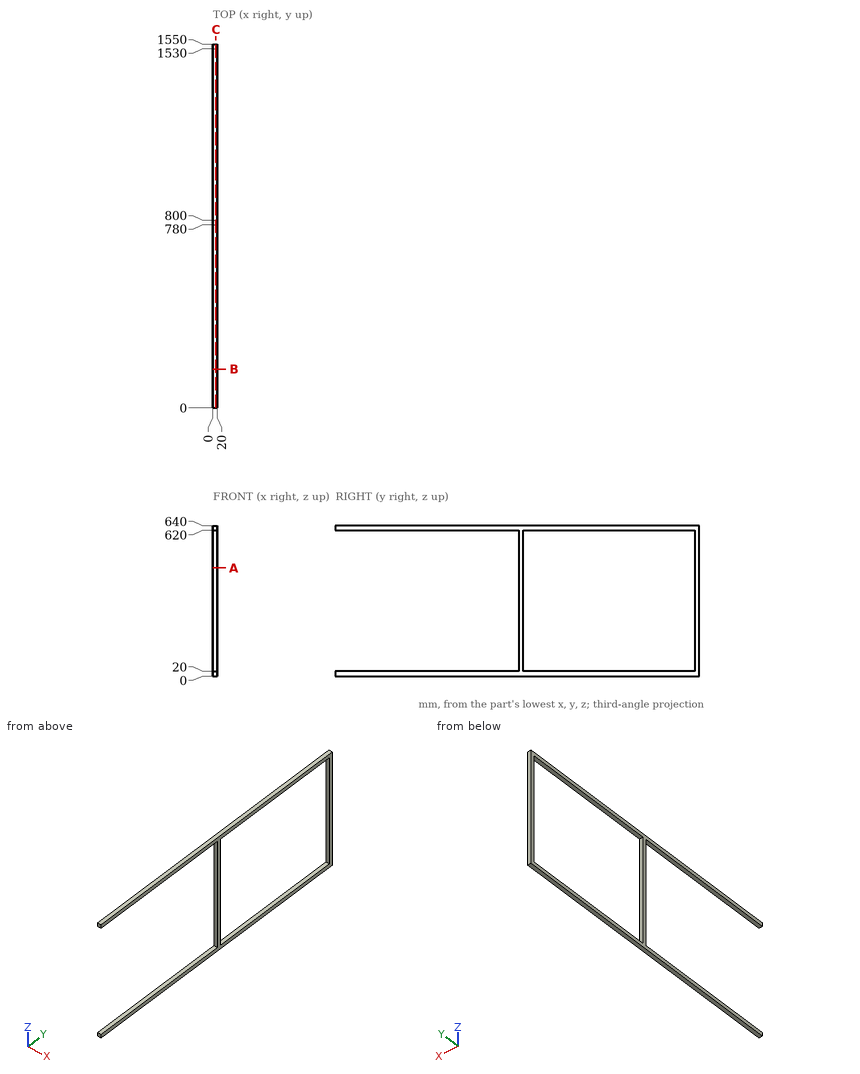
Design review of the part shown in the three views and the two pictorial views. Dimensions are in mm from the part's minimum x, y and z. Give positions to 0.01 mm unless a question says otherwise; leave off trailing zeros. Write each loop counter-clockwise with the first axis right and the second up, starting at its lowest first coordinate (ties: lowest second). Pieces come first, ordered by that corner, then holes. Notation, with made-up numbers: (-8, -27.75) -> (47, -27.75) arc R22 cw to (47, 11.25) -> close; hole circle Ø3 at (-26.5, 2). An arc over 180 degrees is marked (long way). Answer in a Markdown table with one row per item.
1) Add section A-A on z = 461. State the section outline as (x, y) points, plus the area to 3 significant figures.
Worked answers:
| item | result |
|---|---|
| outline | (0, 780) -> (20, 780) -> (20, 800) -> (0, 800) -> close; (0, 1530) -> (20, 1530) -> (20, 1550) -> (0, 1550) -> close |
| area | 800 mm² |
2) For L1, parallel to Y at x = 4, z = 430; L2, parallel to Z at x = 4.25, y = 1110, list the stretches that pass through material, from the lowest coordinate up. Write a range as [from, to].
Worked answers:
| item | result |
|---|---|
| L1 | [780, 800], [1530, 1550] |
| L2 | [0, 20], [620, 640] |
3) Add section C-C on x = 13.75. State the section outline as (y, z) points, plus the area to 3 significant figures.
Worked answers:
| item | result |
|---|---|
| outline | (0, 0) -> (1550, 0) -> (1550, 640) -> (0, 640) -> (0, 620) -> (780, 620) -> (780, 20) -> (0, 20) -> close; hole (800, 20) -> (1530, 20) -> (1530, 620) -> (800, 620) -> close |
| area | 86,000 mm² |
4) Add section B-B on y = 165. State the section outline as (x, z) points, plus the area to 3 significant figures.
Worked answers:
| item | result |
|---|---|
| outline | (0, 0) -> (20, 0) -> (20, 20) -> (0, 20) -> close; (0, 620) -> (20, 620) -> (20, 640) -> (0, 640) -> close |
| area | 800 mm² |
5) Clearance check with flat-ended pins moving along their axes: P1, Ø12, axis at x = 15, z = 130.5, coming from the -Y side; P2, Ø6, axis at x = 13.5, y = 1112, coming from the -Z side. State where each tip first meets the part, or that it passes through.
Worked answers:
| item | result |
|---|---|
| P1 | y = 780 |
| P2 | z = 0 |
